Can you work these out from the drawing? Everything is in mm from the part's minimum corner. Give positions to 0.01 mm unless a question says otherwise; leave off trailing zeros. Order: outer loops, then holes, each group sorted by start corner. A loop starts at its lowest first (then second) coordinate and runs counter-clockwise, first axis right, second up. Notation, with made-up numbers: (2.25, 63.5) - (30.25, 63.5) arc R22 cw to (30.25, 72.5) - close; hole circle Ø5 at (64, 67). An arc over 180 degrees is marked (long way). One line per question, with ' | ' between items.
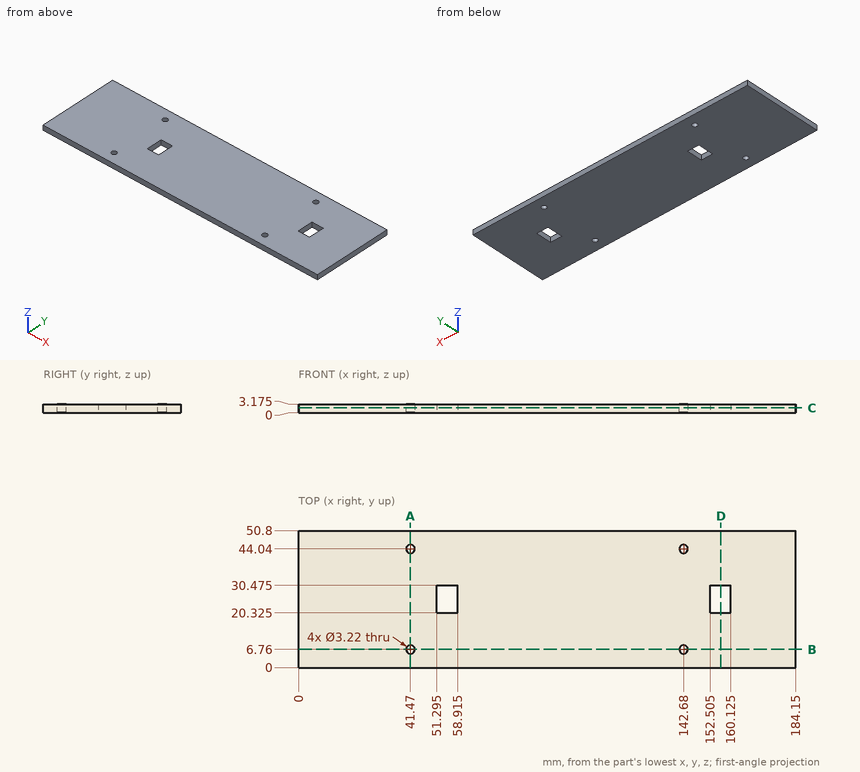
1) I want a section at A-A (x = 41.47). List the corners of the cut face in (y, z) for me (3 decimals).
Model answer:
outline: (0, 0) - (5.15, 0) - (5.15, 3.175) - (0, 3.175) - close; (8.37, 0) - (42.43, 0) - (42.43, 3.175) - (8.37, 3.175) - close; (45.65, 0) - (50.8, 0) - (50.8, 3.175) - (45.65, 3.175) - close
2) I'm going to push a flat-ended pin straight in: P1, Ø3, axis at x = 136, y = 18, coming from the -Z side. Where does the tip first touch, or does it pass through?
Model answer:
P1: stops at z = 0
3) I want a section at C-C (z = 1.7). List the corners of the cut face in (x, y) for me (3 decimals).
Model answer:
outline: (0, 0) - (184.15, 0) - (184.15, 50.8) - (0, 50.8) - close; hole circle Ø3.22 at (41.47, 6.76); hole circle Ø3.22 at (41.47, 44.04); hole (51.295, 20.325) - (58.915, 20.325) - (58.915, 30.475) - (51.295, 30.475) - close; hole circle Ø3.22 at (142.68, 6.76); hole circle Ø3.22 at (142.68, 44.04); hole (152.505, 20.325) - (160.125, 20.325) - (160.125, 30.475) - (152.505, 30.475) - close
4) I want a section at D-D (x = 156.5). List the corners of the cut face in (y, z) for me (3 decimals), plus the area to 3 significant figures.
Model answer:
outline: (0, 0) - (20.325, 0) - (20.325, 3.175) - (0, 3.175) - close; (30.475, 0) - (50.8, 0) - (50.8, 3.175) - (30.475, 3.175) - close | area: 129 mm2
5) I want a section at B-B (y = 6.76). List the corners of the cut face in (x, z) for me (3 decimals).
Model answer:
outline: (0, 0) - (39.86, 0) - (39.86, 3.175) - (0, 3.175) - close; (43.08, 0) - (141.07, 0) - (141.07, 3.175) - (43.08, 3.175) - close; (144.29, 0) - (184.15, 0) - (184.15, 3.175) - (144.29, 3.175) - close
6) Please list where these lines run through material, in increasing order: L1, parallel to Y at x = 142.68, z = 1.85; L2, parallel to X at y = 30, z = 2.05 (3 decimals); L3, parallel to X at y = 43, z = 1.9.
Model answer:
L1: y = 0 to 5.15, 8.37 to 42.43, 45.65 to 50.8 | L2: x = 0 to 51.295, 58.915 to 152.505, 160.125 to 184.15 | L3: x = 0 to 40.24, 42.7 to 141.45, 143.91 to 184.15
